from build123d import *

# Parameters (mm, degrees)
BOSS_EXTRUDE1_DEPTH      = 225
BOSS_EXTRUDE1_DEPTH_BACK = 110
SKETCH1_W                = 10
SKETCH1_H                = 20
SKETCH1_W_2              = 8
SKETCH1_H_2              = 18
SKETCH2_R                = 2.5
CUT_EXTRUDE1_DEPTH       = 1
SKETCH3_R                = 2.5
CUT_EXTRUDE2_DEPTH       = 20


with BuildPart() as part:
    # Sketch1 → Boss-Extrude1 (new, two sides: drawn at the far end of the back side and taken through both)
    with BuildSketch(Plane(origin=(0, 0, 0), x_dir=(0, 0, -1), z_dir=(1, 0, 0)).offset(-BOSS_EXTRUDE1_DEPTH_BACK)):
        Rectangle(SKETCH1_W, SKETCH1_H)
        Rectangle(SKETCH1_W_2, SKETCH1_H_2, mode=Mode.SUBTRACT)
    extrude(amount=BOSS_EXTRUDE1_DEPTH + BOSS_EXTRUDE1_DEPTH_BACK)

    # Sketch2 → Cut-Extrude1 (cut)
    with BuildSketch(Plane.XY.offset(5)):
        with Locations((-19.85, 0)):
            Circle(SKETCH2_R)
        with Locations((-10, 0)):
            Circle(SKETCH2_R)
        Circle(SKETCH2_R)
        with Locations(Location((19.85, 0, 0), (0, 0, 180))):
            Circle(SKETCH2_R)
        with Locations(Location((10, 0, 0), (0, 0, 180))):
            Circle(SKETCH2_R)
    extrude(amount=-CUT_EXTRUDE1_DEPTH, mode=Mode.SUBTRACT)

    # Sketch3 → Cut-Extrude2 (cut)
    with BuildSketch(Plane(origin=(0, 10, 0), x_dir=(1, 0, 0), z_dir=(0, 1, 0))):
        with Locations(Location((220, 0, 0), (0, 0, 270))):
            Circle(SKETCH3_R)
        with Locations(Location((-105, 0, 0), (0, 0, 270))):
            Circle(SKETCH3_R)
    extrude(amount=-CUT_EXTRUDE2_DEPTH, mode=Mode.SUBTRACT)


solid = part.part
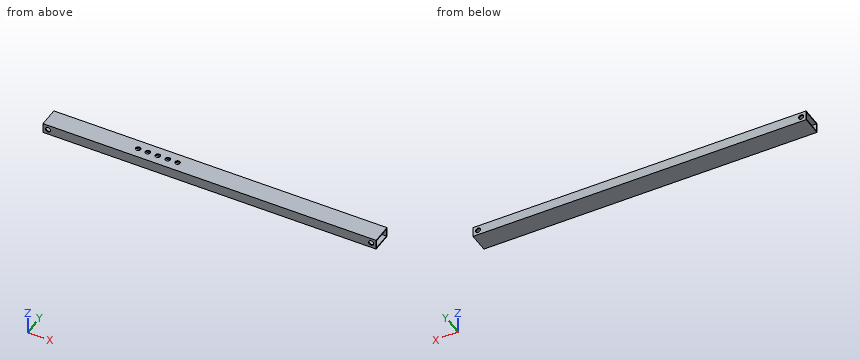
Could you check a few things on this model? Use its own coordinates, in mm. Give positions to 0.01 mm unless a question says otherwise; leave off trailing zeros. Write each loop counter-clockwise with the first axis right and the second up, starting at its lowest first coordinate (ties: lowest second). Pieces come first, ordered by that corner, then holes. Notation, with made-up numbers: (-25, 21) -> (-18, 21) arc R24 cw to (-18, 52) -> close; hole circle Ø10 at (32, 75). An arc over 180 degrees is marked (long way). Write each question's results on one line, items separated by ' | '. Start each with the question number.
Q1. Suppose I cut it at B-B, the plane x = 57. List the corners of the cut face in (y, z) for me.
Q2. Suppose I cut it at A-A, the plane z = 0. List the corners of the cut face in (x, y) for me, and give its area (3 significant figures).
Q3. I need wall thicknesses on probe 1 along X at (y, z) = (-9.35, 0); probe 2 along Y at (x, z) = (197, -3.75); probe 3 along Z at (x, y) = (-70, 8.5). Which ranges of each line are inside material? Lowest first, please.
Q4. I'm going to push flat-ended pins straight in: pin 1 Ø4.5 at (x, y) = (-10, 0) entering from +Z; pin 2 Ø4.5 at (x, z) = (-105, 0) entering from -Y. Where does each tip first touch, or does it pass through?
Outcome:
1) outline: (-10, -5) -> (10, -5) -> (10, 5) -> (-10, 5) -> close; hole (-9, -4) -> (9, -4) -> (9, 4) -> (-9, 4) -> close
2) outline: (-110, -10) -> (-107.5, -10) -> (-107.5, -9) -> (-110, -9) -> close; (-110, 9) -> (-107.5, 9) -> (-107.5, 10) -> (-110, 10) -> close; (-102.5, -10) -> (217.5, -10) -> (217.5, -9) -> (-102.5, -9) -> close; (-102.5, 9) -> (217.5, 9) -> (217.5, 10) -> (-102.5, 10) -> close; (222.5, -10) -> (225, -10) -> (225, -9) -> (222.5, -9) -> close; (222.5, 9) -> (225, 9) -> (225, 10) -> (222.5, 10) -> close | area: 650 mm2
3) probe 1: -110 to -107.5, -102.5 to 217.5, 222.5 to 225 | probe 2: -10 to -9, 9 to 10 | probe 3: -5 to -4, 4 to 5
4) pin 1: z = -4 | pin 2: through
